Input: part model. Units: mm. Frame: model coordinates. A direction names the side the tool comes from. Coordinates: 2 decimals unless noted, no trailing zeros. Order: outer loops, then holes, each group sorted by start corner. A loop starts at its lowest first (then second) coordinate and runs counter-clockwise, first axis right, second up. Notation, with made-up numbers: (71, 22) - (108, 22) arc R18 ccw to (108, 26) - close; hole circle Ø4 at (45.25, 53). An arc over 180 degrees is marked (long way). Answer as CSV lines item,"result". Start each with the question number.
Item 1: First-contact query: pin 1 (1.5 mm diameter, centred on x = -78, z = 94, fed in from -Y); pin 2 (5 mm diameter, centred on x = 89, y = -64, fed in from +Z); pin 3 (8 mm diameter, centred on x = -36.5, z = 154, fed in from -Y). Flat tips, straight axial feed; report the tip coordinate or a pass-through.
Item 2: Access query for faces 1 (the flat face through (3, -71, 0)), 2 (the flat face through (2.93, -90.65, 137.8)). Directions: +Z, -Z, +X, -X, +Y, -Y. A direction counts if a zero-diameter tool reaches every point of the face in a straight line with its end or side. Return the directions, or none.
Item 3: Section B-B (x = 76). Output: boundary loops of the cut face in (y, z), and give its area (3 significant figures).
Item 4: Section A-A (y = -105.5). Output: boundary loops of the cut face in (x, z), and give its area (3 significant figures).
Item 5: Section D-D (z = 168.5). Output: boundary loops of the cut face in (x, y), and give its area (3 significant figures).
Item 6: Draft query along X for faces 3 (the flat face through (-209.55, -71, 54)), 4 (the flat face through (3, -69, 88.9)), 5 (the flat face through (-133.412, -86.4, 142.3)). Return one class per face: +X half, -X half, draft (parallel to the pull), parting line (faces both ways), or undercut.
Item 7: Section C-C (y = -35.5). Output: boundary loops of the cut face in (x, z).
Item 8: Material intervals for line 1 along Z through (x, y) = (135, -15); line 2 along Z through (x, y) = (-81.5, -41); line 3 along Z through (x, y) = (143.5, -51.5), sorted ascending.
from build123d import *

# Parameters (mm, degrees)
F1_DEPTH = 209.55
F2_W     = 26.19375
F2_H     = 26.19375
F3_DEPTH = 0.4064


# Not quite as in the source:
# - the dataset's text gives a spline's control points without its knots; the knots are read off the source's solid


with BuildPart() as f1:
    # F0 (on Right) → F1 (new body, symmetric)
    with BuildSketch(Plane.YZ):
        Polygon((-139.7, 0), (0, 0), (0, 88.9), (-139.2936, 88.9), (-139.2936, 89.154), (-40.6298144724, 187.8177855276), (-40.9171826682, 188.1051537235), (-139.7, 89.3223363917), align=None)
    extrude(amount=F1_DEPTH, both=True)

    # F2 (on face) → F3 (cut, through all)
    with BuildSketch(Plane(origin=(0, -114.5111681959, 114.5111681959), x_dir=(1, 0, 0), z_dir=(0, -0.7071067812, 0.7071067812))):
        with Locations((-146.5093133926, 39.7379171954)):
            Rectangle(F2_W, F2_H)
        with BuildLine():
            add(Edge.make_bspline(
                [(168.6742066074, 50.1214371954), (165.9556700074, 52.8397705954), (162.1350528074, 54.4222921954), (158.2906866074, 54.4222921954)],
                knots=[7, 7, 7, 7, 8, 8, 8, 8], degree=3))
            add(Edge.make_bspline(
                [(158.2906866074, 54.4222921954), (154.4462950074, 54.4222921954), (150.6256778074, 52.8397705954), (147.9074968074, 50.1214371954)],
                knots=[0, 0, 0, 0, 1, 1, 1, 1], degree=3))
            add(Edge.make_bspline(
                [(147.9074968074, 50.1214371954), (145.1889856074, 47.4029005954), (143.6063116074, 43.5822833954), (143.6063116074, 39.7379171954), (143.6063116074, 35.8935255954), (145.1889856074, 32.0729083954), (147.9074968074, 29.3543971954)],
                knots=[1, 1, 1, 1, 2, 2, 2, 3, 3, 3, 3], degree=3))
            add(Edge.make_bspline(
                [(147.9074968074, 29.3543971954), (150.6256778074, 26.6360383954), (154.4462950074, 25.0535421954), (158.2906866074, 25.0535421954), (162.1350528074, 25.0535421954), (165.9556700074, 26.6360383954), (168.6742066074, 29.3543971954)],
                knots=[3, 3, 3, 3, 4, 4, 4, 5, 5, 5, 5], degree=3))
            add(Edge.make_bspline(
                [(168.6742066074, 29.3543971954), (171.3927178074, 32.0729083954), (172.9750616074, 35.8935255954), (172.9750616074, 39.7379171954), (172.9750616074, 43.5822833954), (171.3927178074, 47.4029005954), (168.6742066074, 50.1214371954)],
                knots=[5, 5, 5, 5, 6, 6, 6, 7, 7, 7, 7], degree=3))
        make_face()
    extrude(amount=-F3_DEPTH, mode=Mode.SUBTRACT)


solid = f1.part
Determined:
1,pin 1,"stops at y = -135.77"
1,pin 2,"stops at z = 167.52"
1,pin 3,"stops at y = -79.02"
2,face 1,"-Z, +X, -X, +Y, -Y"
2,face 2,"+X, -X, +Y"
3,outline,"(-139.7, 0) - (0, 0) - (0, 88.9) - (-139.29, 88.9) - (-139.29, 89.15) - (-40.63, 187.82) - (-40.92, 188.11) - (-139.7, 89.32) - close"
3,area,"12,500 mm^2"
4,outline,"(-209.55, 0) - (209.55, 0) - (209.55, 88.9) - (-209.55, 88.9) - close; (-209.55, 122.95) - (209.55, 122.95) - (209.55, 123.52) - (-209.55, 123.52) - close"
4,area,"37,500 mm^2"
5,outline,"(-209.55, -60.52) - (209.55, -60.52) - (209.55, -59.95) - (-209.55, -59.95) - close"
5,area,"241 mm^2"
6,face 3,"-X half"
6,face 4,"draft"
6,face 5,"undercut"
7,outline,"(-209.55, 0) - (209.55, 0) - (209.55, 88.9) - (-209.55, 88.9) - close"
8,line 1,"z = 0 to 88.9"
8,line 2,"z = 0 to 88.9, 187.45 to 188.02"
8,line 3,"z = 0 to 88.9, 176.95 to 177.52"
